Build history of the part. All positions in model axes, mm. A direction names the side the tool comes from. Round coordinates to 2 decimals unless told otherwise and drop trailing zeros. Order: outer loops, then holes, each group sorted by start corner. A loop starts at its lowest first (then second) coordinate and runs counter-clockwise, first axis right, second up. Notation, with made-up numbers: (-18.75, 28) -> (14.25, 28) arc R20 cw to (14.25, 33) -> close; hole circle Ø9 at (-13.75, 56). An arc over 180 degrees is marked (long way). Write item = value, one per line.
from build123d import *

# Parameters (mm, degrees)
SALIENTE_EXTRUIR1_DEPTH = 5.5
CORTAR_EXTRUIR1_DEPTH   = 5.5
CORTAR_EXTRUIR4_DEPTH   = 5.5
CORTAR_EXTRUIR5_DEPTH   = 5.5


with BuildPart() as part:
    # Croquis1 → Saliente-Extruir1 (new body)
    with BuildSketch(Plane.XY):
        Polygon((180, 0), (180, 93.289473684), (274.896352923, 138.268626086), (210.65044876, 273.81368796), (-42.36700007, 153.888000188), (15.880022719, 30.999289839), (-13.188895459, 17.615531012), (-40.600481236, 75.448090745), (-60, 75.448090745), (-60, 0), (-26, 0), (-26, 5.5), (8.66, 5.5), (8.66, 0), (42.66, 0), (42.66, 5.5), (77.34, 5.5), (77.34, 0), (111.34, 0), (111.34, 5.5), (146, 5.5), (146, 0), align=None)
    extrude(amount=SALIENTE_EXTRUIR1_DEPTH)

    # Croquis2 → Cortar-Extruir1 (cut)
    with BuildSketch(Plane.XY.offset(5.5)):
        Polygon((180, 93.289473684), (57.917117024, 35.663353874), (60.264847831, 30.68960679), (180, 87.207539986), align=None)
    extrude(amount=-CORTAR_EXTRUIR1_DEPTH, mode=Mode.SUBTRACT)

    # Croquis4 → Cortar-Extruir4 (cut)
    with BuildSketch(Plane.XY.offset(5.5)):
        Polygon((-43.332939479, 56.464331481), (-38.272590503, 58.862845236), (-33.989530225, 49.826507778), (-39.049879202, 47.427994023), align=None)
        Polygon((-35.409277966, 39.747107183), (-30.348928989, 42.145620939), (-26.065868712, 33.10928348), (-31.126217688, 30.710769725), align=None)
        Polygon((-27.485616452, 23.029882886), (-22.425267476, 25.428396641), (-18.142207198, 16.392059183), (-23.202556175, 13.993545427), align=None)
    extrude(amount=-CORTAR_EXTRUIR4_DEPTH, mode=Mode.SUBTRACT)

    # Croquis5 → Cortar-Extruir5 (cut)
    with BuildSketch(Plane.XY.offset(5.5)):
        Polygon((25.170422415, 174.833084673), (27.526105568, 169.863099071), (45.598780484, 178.429219626), (43.243097332, 183.399205228), align=None)
        Polygon((133.606471914, 226.229808004), (151.67914683, 234.795928559), (154.034829983, 229.825942957), (135.962155066, 221.259822402), align=None)
    extrude(amount=-CORTAR_EXTRUIR5_DEPTH, mode=Mode.SUBTRACT)


solid = part.part
Q1. Cut at D-D, the plane y = 202. List the corners of the cut face in (x, z).
Check values:
outline = (59.14, 0) -> (244.69, 0) -> (244.69, 5.5) -> (59.14, 5.5) -> close
Q2. Probe probe 1 along X at (y, z) = (18, 3.2); probe 2 along Y at (x, z) = (153, 4.3); probe 3 along Y at (x, z) = (-13.5, 1.85). List the from-to ranges inside material, lowest first.
Check values:
probe_1 = -60 to -25.1, -18.9 to -13.37, -12.35 to 180
probe_2 = 0 to 74.46, 80.54 to 229.34, 232.01 to 246.49
probe_3 = 5.5 to 18.27, 92.98 to 167.57
Q3. Cut at B-B, the plane z = 1.1. Give the number of separate pieces and of enclosed holes in the cut face, and give its area (3 significant figures).
Check values:
separate_pieces = 1
enclosed_holes = 5
area = 52,700 mm²
Q4. Cut at A-A, the plane x = 70.5. List the corners of the cut face in (y, z).
Check values:
outline = (5.5, 0) -> (35.52, 0) -> (35.52, 5.5) -> (5.5, 5.5) -> close; (41.6, 0) -> (207.38, 0) -> (207.38, 5.5) -> (41.6, 5.5) -> close
Q5. Which spindle directions (+Z, -Z, +X, -X, +Y, -Y) get a long thin tool onto all of the face, cutting with end or side? Do faces 4 (the face through (105, 108, 5.5)), 5 (the face through (145.125, 225.603, 2.788)). Say none if no direction does.
Check values:
face_4 = +Z, +X, -X, +Y, -Y
face_5 = +Z, -Z
Q6. Cut at C-C, the plane x = 163.5. List the corners of the cut face in (y, z), and give its area (3 significant figures).
Check values:
outline = (0, 0) -> (79.42, 0) -> (79.42, 5.5) -> (0, 5.5) -> close; (85.5, 0) -> (251.47, 0) -> (251.47, 5.5) -> (85.5, 5.5) -> close
area = 1,350 mm²
Q7. Mould opens along Y. For faces 1 (the face through (226.784, 115.464, 2.712)), 2 (the face through (-26.703, 46.127, 2.712)), 3 (the face through (85.91, 214.69, 2.71)) say: released by +Y, released by -Y, zero draft, split by the parting line, or undercut.
Check values:
face_1 = released by -Y
face_2 = undercut
face_3 = released by +Y
Q8. Flat gauge pins, fed straight in: pin 1 (1.5 mm diameter, centred on y = 161, z = 2, fed in from -X); pin 2 (1.6 mm diameter, centred on x = 132.5, z = 2.5, fed in from -Y); pin 3 (8 mm diameter, centred on x = 8.5, y = 30.5, fed in from -Z); pin 4 (2 mm diameter, centred on y = 214, z = 3, fed in from +X). Where does each tip first touch, or does it go through?
Check values:
pin_1 = -28.94
pin_2 = 5.5
pin_3 = 0
pin_4 = 239.48
